```python
from build123d import *

# Parameters (mm, degrees)
SKETCH1_R             = 2.5
BOSS_EXTRUDE3_DEPTH   = 3.5
F_6_0MM_DOWEL_HOLE4_D = 6


with BuildPart() as part:
    # Sketch1 → Boss-Extrude3 (new body)
    with BuildSketch(Plane(origin=(0, 0, 0), x_dir=(1, 0, 0), z_dir=(0, 1, 0))):
        with BuildLine():
            Line((-18.084732229, -7.982467334), (229.915267771, -7.982467334))
            ThreePointArc((229.915267771, -7.982467334), (251.128471207, 0.80432923), (259.915267771, 22.017532666))
            Line((259.915267771, 22.017532666), (259.915267771, 39.017532666))
            ThreePointArc((259.915267771, 39.017532666), (251.128471207, 60.230736102), (229.915267771, 69.017532666))
            Line((229.915267771, 69.017532666), (31.915267771, 69.017532666))
            Line((31.915267771, 69.017532666), (31.915267771, 65.517532666))
            Line((31.915267771, 65.517532666), (31.915267771, 52.017532666))
            Line((31.915267771, 52.017532666), (-18.084732229, -7.982467334))
        make_face()
        with Locations(Location((149.915267771, 30.517532666, 0), (0, 0, 270))):
            Circle(SKETCH1_R, mode=Mode.SUBTRACT)
        with Locations(Location((109.915267771, 30.517532666, 0), (0, 0, 270))):
            Circle(SKETCH1_R, mode=Mode.SUBTRACT)
        with Locations(Location((69.915267771, 30.517532666, 0), (0, 0, 270))):
            Circle(SKETCH1_R, mode=Mode.SUBTRACT)
    extrude(amount=BOSS_EXTRUDE3_DEPTH)

    # Ø6.0mm Dowel Hole4 (through all)
    with Locations(Plane(origin=(224.539982251, 261.5, -21.544477375), x_dir=(1, 0, 0), z_dir=(0, 1, 0))):
        with Locations((-95.797211751, -5.414641336)):
            Hole(F_6_0MM_DOWEL_HOLE4_D / 2)


solid = part.part
```
Verification items for the finished model (mm, model axes). Round coordinates to 2 decimals unless told otherwise and drop trailing zeros. Write each loop counter-clockwise with the first axis right and the second up, starting at its lowest first coordinate (ties: lowest second). Pieces come first, ordered by that corner, then holes. Notation, with made-up numbers: (18.25, 69) - (49.25, 69) arc R33 ccw to (49.25, 100) - close; hole circle Ø1 at (50, 28.5). An arc over 180 degrees is marked (long way). Answer as a JSON object with one key per item and string values. Group by question number.
Q1. Section check B-B, the plane z = -4.5. Enter the section's corners in (x, y).
Q2. Mould release check, pull along X, two halves, no side actions. Record for faces 1 (the flat face through (119, 0, -31)), 2 (the cylindrical face through (250.89, 1.73, -0.57)), 3 (the cylindrical face through (112.4, 1.7, -30.8)): released by +X, released by -X, zero draft, split by the parting line, or undercut.
Q3. Section check C-C, the plane z = -45. Enter the section's corners in (x, y), plus the area to 3 significant figures.
Q4. Go/stop test with flat-tipped pins: pin 1 Ø6.5 at (x, z) = (69.92, -30.52) entering from +Y; pin 2 Ø1.8 at (y, z) = (1.5, -56.5) entering from -X. Record where each tip stops, or that it passes through.
Q5. Section check A-A, the plane y = 1.5. Enter the section's corners in (x, z), plus the area to 3 significant figures.
Q6. Thickness scan on line 1 (X direction, y = 1.3, z = -32.5); line 2 (X direction, y = 2.45, z = -14); line 3 (Z direction, x = 235.5, y = 2.1). Record the ranges inside material, lowest first.
Found:
{
 "1": {"outline": "(-7.68, 0) - (254.27, 0) - (254.27, 3.5) - (-7.68, 3.5) - close"},
 "2": {"face 1": "zero draft", "face 2": "released by +X", "face 3": "undercut"},
 "3": {"outline": "(26.07, 0) - (259.31, 0) - (259.31, 3.5) - (26.07, 3.5) - close", "area": "816 mm^2"},
 "4": {"pin 1": "stops at y = 3.5", "pin 2": "stops at x = 31.92"},
 "5": {"outline": "(-18.08, 7.98) - (31.92, -52.02) - (31.92, -69.02) - (229.92, -69.02) arc R30 ccw to (259.92, -39.02) - (259.92, -22.02) arc R30 ccw to (229.92, 7.98) - close; hole circle Ø5 at (69.92, -30.52); hole circle Ø5 at (109.92, -30.52); hole circle Ø6 at (128.74, -16.13); hole circle Ø5 at (149.92, -30.52)", "area": "18,600 mm^2"},
 "6": {"line 1": "x = 15.65 to 68.39, 71.44 to 108.39, 111.44 to 148.39, 151.44 to 259.92", "line 2": "x = 0.23 to 126.63, 130.86 to 258.82", "line 3": "z = -68.49 to 7.46"}
}
